Source: three-view drawing plus pictorial views. Frame: mm from the lowest corner of the part. Coordinates: 2 decimals unless noted, no trailing zeros. Order: outer loops, then holes, each group sorted by start corner. A loop starts at its lowest first (then second) coordinate and runs counter-clockwise, first axis right, second up. Notation, with made-up numbers: M 88.5,18 L 130.5,18 A17 cw 130.5,36 Z; hole C 77,-31.5 d9. An arc over 180 degrees is marked long. Write item = value, one per line. Start each with the question number.
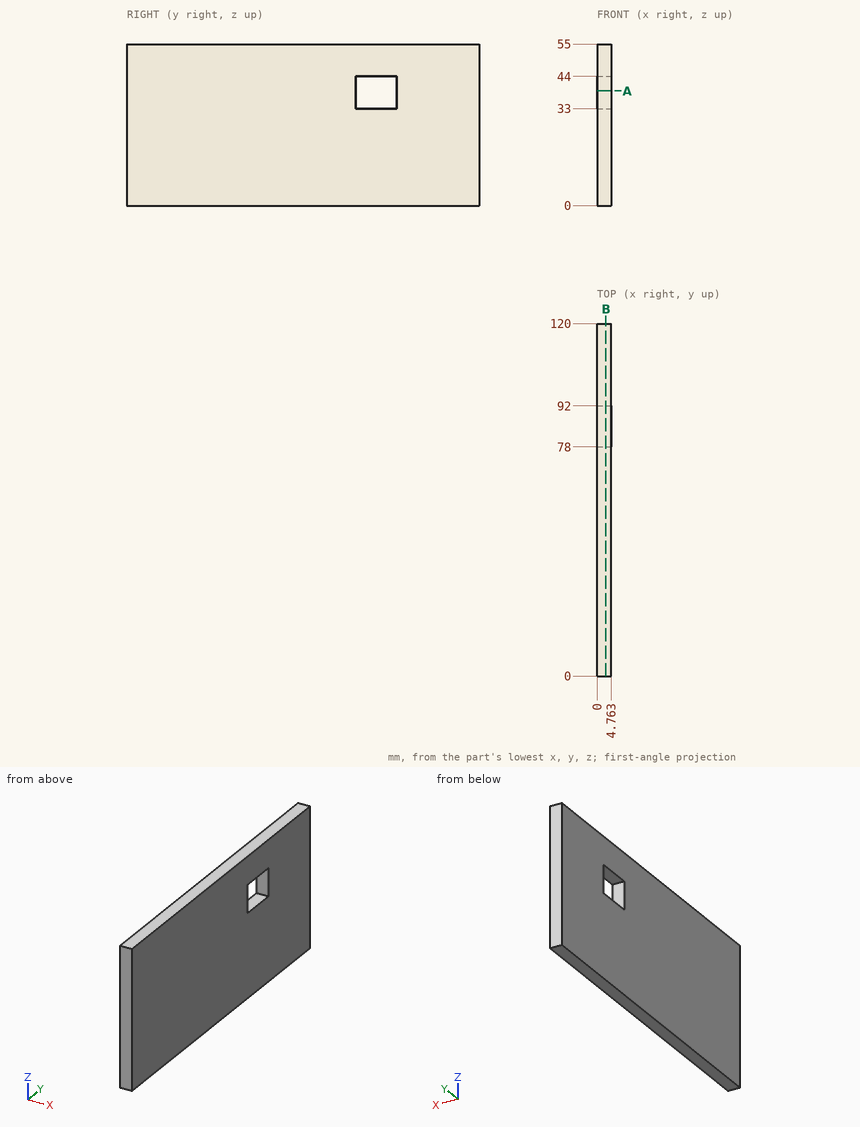
Item 1: Material intervals for probe 1 along Y at (x, z) = (2, 36); probe 2 along Z at (x, y) = (0.5, 82), sorted ascending. Write a range as [from, to].
Item 2: Section query A-A on z = 39. Output: boundary loops of the cut face in (x, y), and give its area (3 significant figures).
Item 3: Section query B-B on x = 2.95. Output: boundary loops of the cut face in (y, z), and give its area (3 significant figures).
Ans:
q1.probe_1 = [0, 78], [92, 120]
q1.probe_2 = [0, 33], [44, 55]
q2.outline = M 0,0 L 4.76,0 L 4.76,78 L 0,78 Z; M 0,92 L 4.76,92 L 4.76,120 L 0,120 Z
q2.area = 505 mm^2
q3.outline = M 0,0 L 120,0 L 120,55 L 0,55 Z; hole M 78,33 L 92,33 L 92,44 L 78,44 Z
q3.area = 6,450 mm^2
